```python
from build123d import *

# Parameters (mm, degrees)
SKETCH1_W           = 16.6
SKETCH1_H           = 16.6
BOSS_EXTRUDE1_DEPTH = 10
SKETCH3_R           = 5
CUT_EXTRUDE1_DEPTH  = 10
SKETCH4_R           = 8.3
SKETCH4_R_2         = 2.5
BOSS_EXTRUDE2_DEPTH = 10


with BuildPart() as part:
    # Sketch1 → Boss-Extrude1 (new body)
    with BuildSketch(Plane(origin=(0, 0, 0), x_dir=(1, 0, 0), z_dir=(0, 1, 0))):
        Rectangle(SKETCH1_W, SKETCH1_H)
    extrude(amount=BOSS_EXTRUDE1_DEPTH)

    # Sketch3 → Cut-Extrude1 (cut)
    with BuildSketch(Plane.XZ):
        with Locations(Location((0, 0, 0), (0, 0, 270))):
            Circle(SKETCH3_R)
    extrude(amount=-CUT_EXTRUDE1_DEPTH, mode=Mode.SUBTRACT)

    # Sketch4 → Boss-Extrude2 (add)
    with BuildSketch(Plane.XZ):
        with Locations(Location((0, 0, 0), (0, 0, 270))):
            Circle(SKETCH4_R)
        with Locations(Location((0, 0, 0), (0, 0, 270))):
            Circle(SKETCH4_R_2, mode=Mode.SUBTRACT)
    extrude(amount=BOSS_EXTRUDE2_DEPTH)


solid = part.part
```
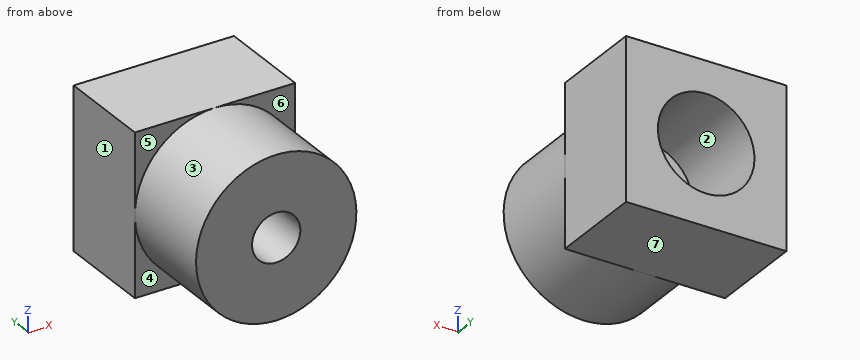
CAD build for the part. Positions are in the model's coordinates, mm. Face numbers are marked on the shaded views. A direction names the side the tool comes from. Round coordinates to 2 decimals unless told otherwise and drop trailing zeros. Order: outer loops, then holes, each group sorted by start corner. A loop starts at its lowest first (then second) coordinate and runs counter-clockwise, first axis right, second up.
Q1. Slice it at C-C (x = 6.75). Write the cut outline in (y, z), and give its area (3 significant figures).
Q2. Slice it at A-A (y = 1). Write the cut outline in (x, z).
Q3. Two-plate mould, pull along Z, no slides. Class the marked faces 1, 2 and 3: pulls with the +Z half, pulls with the -Z half, needs draft (parallel to the pull), parting line crosses it, or undercut.
Q4. Slice it at D-D (z = -2.25). Write the cut outline in (x, y), and give its area (3 significant figures).
Q5. Which spindle directions (+Z, -Z, +X, -X, +Y, -Y) get a long thin tool onto all of the face, cutting with end or side? Do the marked faces 4, 5, 6 and 7. Say none if no direction does.
Q6. Drop flat-ended pins along their axis: pin 1 (1 mm diameter, centred on y = -1, z = -2.5, fed in from +X); pin 2 (1.5 mm diameter, centred on x = -5, y = -8, fed in from -Z); pin 3 (5 mm diameter, centred on x = 1, z = 1, fed in from +Y). Give the stop position or say it passes through.
Q7. Wall check: L1, parallel to X at y = 4.75, z = 0; L2, parallel to X at y = -6.5, z = 0; L3, parallel to Y at x = 1.5, z = -4.25. Give the ranges that are in metal, low to high.
Results below:
1. outline: (-10, -4.83) - (0, -4.83) - (0, -8.3) - (10, -8.3) - (10, 8.3) - (0, 8.3) - (0, 4.83) - (-10, 4.83) - close
1. area: 263 mm2
2. outline: (-8.3, -8.3) - (8.3, -8.3) - (8.3, 8.3) - (-8.3, 8.3) - close; hole circle Ø10 at (0, 0)
3. face 1: needs draft
3. face 2: undercut
3. face 3: parting line crosses it
4. outline: (-8.3, 0) - (-7.99, 0) - (-7.99, -10) - (-1.09, -10) - (-1.09, 0) - (-4.47, 0) - (-4.47, 10) - (-8.3, 10) - close; (1.09, -10) - (7.99, -10) - (7.99, 0) - (8.3, 0) - (8.3, 10) - (4.47, 10) - (4.47, 0) - (1.09, 0) - close
4. area: 215 mm2
5. face 4: -Z, -X, -Y
5. face 5: +Z, -X, -Y
5. face 6: +Z, +X, -Y
5. face 7: -Z, +X, -X, +Y, -Y
6. pin 1: stops at x = 8.06
6. pin 2: stops at z = -7.13
6. pin 3: stops at y = 0
7. L1: x = -8.3 to -5, 5 to 8.3
7. L2: x = -8.3 to -2.5, 2.5 to 8.3
7. L3: y = -10 to 0
